The model under review builds one solid part; all positions refer to its coordinate system, in mm. Face numbers are marked on the shaded views. Coordinates: 2 decimals unless noted, no trailing zeros. Write each loop counter-clockwise with the first axis right and the second up, starting at its lowest first coordinate (ties: lowest second). Pieces come first, ordered by that corner, then holes. Notation, with made-up numbers: (88.5, -15.75) -> (100.5, -15.75) arc R30 cw to (100.5, 15.25) -> close; hole circle Ø11 at (16, 79). An arc over 180 degrees is marked (long way). Put each result on its own line as item: value. Start each with the question number.
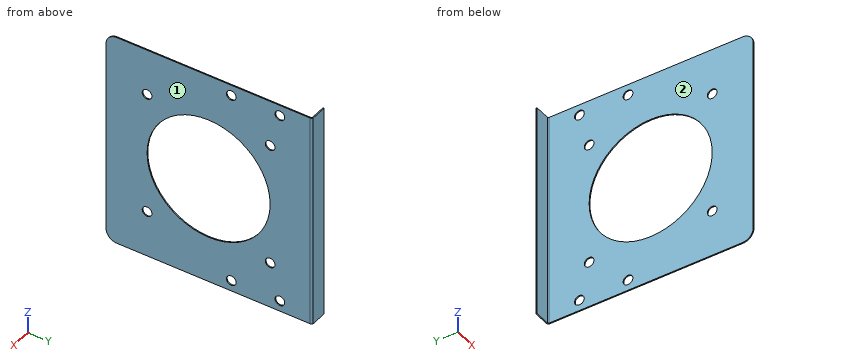
from build123d import *

# Parameters (mm, degrees)
CROQUIS1_R                       = 57
SALIENTE_EXTRUIR1_DEPTH          = 15
VACIADO1_T                       = 1
DESPLEGAR_PLIEGUES1_OUTLINE_W    = 1
DESPLEGAR_PLIEGUES1_OUTLINE_H    = 200
DESPLEGAR_PLIEGUES1_DEPTH        = 15
DESPLEGAR_START                  = 15
DESPLEGAR_PLIEGUES1_2_OUTLINE_W  = 14.35619449
DESPLEGAR_PLIEGUES1_2_OUTLINE_H  = 200
DESPLEGAR_PLIEGUES1_2_DEPTH      = 1
PROCESAR_START                   = -100
PROCESAR_PLIEGUES1_DEPTH         = 200
PROCESAR_PLIEGUES1_2_DEPTH       = 200
TALADRO_DE_MARGEN_PARA_M83_D     = 9
TALADRO_DE_MARGEN_PARA_M84_D     = 9
TALADRO_DE_MARGEN_PARA_M84_DEPTH = 15.42
TALADRO_DE_MARGEN_PARA_M85_D     = 9
TALADRO_DE_MARGEN_PARA_M85_DEPTH = 1.999


# Read off the part's stored shape, not the designer's step: Desplegar pliegues1, Procesar pliegues1
with BuildPart() as part:
    # Croquis1 → Saliente-Extruir1 (new body)
    with BuildSketch(Plane(origin=(0, 0, 0), x_dir=(0, 0, -1), z_dir=(1, 0, 0))):
        with BuildLine():
            Line((-100, 0), (100, 0))
            Line((100, 0), (100, -180))
            ThreePointArc((100, -180), (97.071067812, -187.071067812), (90, -190))
            Line((90, -190), (-90, -190))
            ThreePointArc((-90, -190), (-97.071067812, -187.071067812), (-100, -180))
            Line((-100, -180), (-100, 0))
        make_face()
        with Locations((0, -95)):
            Circle(CROQUIS1_R, mode=Mode.SUBTRACT)
    extrude(amount=SALIENTE_EXTRUIR1_DEPTH)

    # Vaciado1
    vaciado1_openings = [part.faces().sort_by_distance(p)[0] for p in [
        (7.5, -90, -100),
        (7.5, -187.071067812, -97.071067812),
        (7.5, -190, 0),
        (7.5, -187.071067812, 97.071067812),
        (7.5, -90, 100),
        (7.5, -95, 57),
        (0, -2.758622845, 0),
    ]]
    offset(amount=VACIADO1_T, openings=vaciado1_openings, kind=Kind.INTERSECTION)

    # Desplegar pliegues1 outline → Desplegar pliegues1 (cut)
    with BuildSketch(Plane.YZ):
        with Locations((0.5, 0)):
            Rectangle(DESPLEGAR_PLIEGUES1_OUTLINE_W, DESPLEGAR_PLIEGUES1_OUTLINE_H)
    extrude(amount=DESPLEGAR_PLIEGUES1_DEPTH, mode=Mode.SUBTRACT)

    # Desplegar pliegues1 2 outline → Desplegar pliegues1 2 (add)
    with BuildSketch(Plane.YZ.offset(DESPLEGAR_START)):
        with Locations((8.178097245, 0)):
            Rectangle(DESPLEGAR_PLIEGUES1_2_OUTLINE_W, DESPLEGAR_PLIEGUES1_2_OUTLINE_H)
    extrude(amount=DESPLEGAR_PLIEGUES1_2_DEPTH)

    # Procesar pliegues1 outline → Procesar pliegues1 (cut)
    with BuildSketch(Plane.XY.offset(PROCESAR_START)):
        with BuildLine():
            Line((15, 15.35619449), (15, 0.732050807))
            ThreePointArc((15, 0.732050807), (15.732050807, 0), (16, -1))
            Line((16, -1), (16, 15.35619449))
            Line((16, 15.35619449), (15, 15.35619449))
        make_face()
    extrude(amount=PROCESAR_PLIEGUES1_DEPTH, mode=Mode.SUBTRACT)

    # Procesar pliegues1 2 outline → Procesar pliegues1 2 (add)
    with BuildSketch(Plane.XY.offset(PROCESAR_START)):
        with BuildLine():
            Line((14, 1), (0, 1))
            Line((0, 1), (0, 0))
            Line((0, 0), (14, 0))
            ThreePointArc((14, 0), (14.707106781, -0.292893219), (15, -1))
            Line((15, -1), (15, 0.732050807))
            ThreePointArc((15, 0.732050807), (14.51763809, 0.931851652), (14, 1))
        make_face()
    extrude(amount=PROCESAR_PLIEGUES1_2_DEPTH)

    # Taladro de margen para M83 (through all)
    with Locations(Plane(origin=(15, -102.41730184, -252.760845032), x_dir=(0, 0, 1), z_dir=(-1, 0, 0))):
        with Locations((162.760845032, 73.414694032), (162.760845032, 28.414694032), (342.760845032, 73.414694032), (342.760845032, 28.414694032)):
            Hole(TALADRO_DE_MARGEN_PARA_M83_D / 2)

    # Taladro de margen para M84
    with Locations(Plane(origin=(15, -102.41730184, -252.760845032), x_dir=(0, 0, 1), z_dir=(-1, 0, 0))):
        with Locations((195.760845032, 64.41730184), (309.760845032, 64.41730184)):
            Hole(TALADRO_DE_MARGEN_PARA_M84_D / 2, depth=TALADRO_DE_MARGEN_PARA_M84_DEPTH)

    # Taladro de margen para M85
    with Locations(Plane(origin=(15, -102.41730184, -252.760845032), x_dir=(0, 0, 1), z_dir=(-1, 0, 0))):
        with Locations((309.760845032, -49.58269816), (195.760845032, -49.58269816)):
            Hole(TALADRO_DE_MARGEN_PARA_M85_D / 2, depth=TALADRO_DE_MARGEN_PARA_M85_DEPTH)


solid = part.part
1. Consider section A-A on y = -95. State the section outline as (x, z) points, then the cut area to 3 significant figures.
2. The part is to be moulded in two halves that separate along X. For the marked faces 1 and 2, say which applies: released by +X, released by -X, zero draft, split by the parting line, or undercut.
3. Consider section D-D on x = 10. State the section outline as (y, z) points.
4. Consider section C-C on y = -48. State the section outline as (x, z) points.
5. Consider section B-B on z = 26. State the section outline as (x, y) points.
6. Insertion check: P1, Ø14.5, axis at y = -38, z = -57, coming from the -X side; P2, Ø5, axis at x = 10.5, z = 38.5, coming from the -Y side. Each pin has a flat end and moves straight along its axis. Give the tip position at first contact, or say it passes through.
7. Wall thickness on line 1 (Y direction, x = 15.7, z = 90); line 2 (Y direction, x = 15.75, z = 90); line 3 (Y direction, x = 13.5, z = 23.5): over which ranges is each line inside the solid? List them lowest first. Write a range as from..to.
Output values:
1. outline: (15, -100) -> (16, -100) -> (16, -57) -> (15, -57) -> close; (15, 57) -> (16, 57) -> (16, 100) -> (15, 100) -> close
1. area: 86.0 mm^2
2. face 1: released by +X
2. face 2: released by -X
3. outline: (0, -100) -> (1, -100) -> (1, 100) -> (0, 100) -> close
4. outline: (15, -100) -> (16, -100) -> (16, -32.25) -> (15, -32.25) -> close; (15, 32.25) -> (16, 32.25) -> (16, 100) -> (15, 100) -> close
5. outline: (0, 0) -> (14, 0) arc R1 cw to (15, -1) -> (15, -44.28) -> (16, -44.28) -> (16, -1) arc R2 ccw to (14, 1) -> (0, 1) -> close; (15, -190) -> (16, -190) -> (16, -145.72) -> (15, -145.72) -> close
6. P1: stops at x = 15
6. P2: stops at y = 0
7. line 1: y = -190..-78.5, -69.5..-33.5, -24.5..0.05
7. line 2: y = -190..-78.5, -69.5..-33.5, -24.5..-0.03
7. line 3: y = 0..1
